```python
from build123d import *

# Parameters (mm, degrees)
SM_BASE_FLANGE_1_DEPTH              = 8
SM_EDGE_FLANGE_1_STRIP_W            = 48
SM_EDGE_FLANGE_1_STRIP_H            = 8
SM_EDGE_FLANGE_1_STRIP_CUT_DEPTH    = 50
SM_EDGE_FLANGE_1_RELIEF_W           = 52
SM_EDGE_FLANGE_1_RELIEF_H           = 4
SM_EDGE_FLANGE_1_RELIEF_CUT_DEPTH   = 8
SM_EDGE_FLANGE_1_STRIP_2_W          = 48
SM_EDGE_FLANGE_1_STRIP_2_H          = 8
SM_EDGE_FLANGE_1_STRIP_CUT_2_DEPTH  = 50
SM_EDGE_FLANGE_1_RELIEF_2_W         = 52
SM_EDGE_FLANGE_1_RELIEF_2_H         = 4
SM_EDGE_FLANGE_1_RELIEF_CUT_2_DEPTH = 8
SM_EDGE_FLANGE_1_DEPTH              = 50
SM_EDGE_FLANGE_1_BEND_DEPTH         = 50


# Sheet-metal steps are written as plain solids
with BuildPart() as part:
    # Sketch 1 → 基体-法兰1 (new body)
    with BuildSketch(Plane(origin=(0, 0, 0), x_dir=(0, 0, -1), z_dir=(1, 0, 0))):
        Polygon((-52.5, 122), (52.5, 122), (114.5, 60), (114.5, 50), (124.5, 50), (124.5, 0), (-124.5, 0), (-124.5, 50), (-114.5, 50), (-114.5, 60), align=None)
    extrude(amount=-SM_BASE_FLANGE_1_DEPTH)

    # 边线-法兰1 strip (across the edge) → 边线-法兰1 strip cut (cut)
    with BuildSketch(Plane(origin=(-8, 0, 124.5), x_dir=(0, 0, -1), z_dir=(0, 1, 0))):
        with Locations((-8, -4)):
            Rectangle(SM_EDGE_FLANGE_1_STRIP_W, SM_EDGE_FLANGE_1_STRIP_H)
    extrude(amount=SM_EDGE_FLANGE_1_STRIP_CUT_DEPTH, mode=Mode.SUBTRACT)

    # 边线-法兰1 relief (on the sheet) → 边线-法兰1 relief cut (cut)
    with BuildSketch(Plane(origin=(-8, 0, 108.5), x_dir=(0, 0, -1), z_dir=(-1, 0, 0))):
        with Locations((-22, -52)):
            Rectangle(SM_EDGE_FLANGE_1_RELIEF_W, SM_EDGE_FLANGE_1_RELIEF_H)
    extrude(amount=-SM_EDGE_FLANGE_1_RELIEF_CUT_DEPTH, mode=Mode.SUBTRACT)

    # 边线-法兰1 strip 2 (across the edge) → 边线-法兰1 strip cut 2 (cut)
    with BuildSketch(Plane(origin=(-8, 50, -124.5), x_dir=(0, 0, 1), z_dir=(0, -1, 0))):
        with Locations((-8, -4)):
            Rectangle(SM_EDGE_FLANGE_1_STRIP_2_W, SM_EDGE_FLANGE_1_STRIP_2_H)
    extrude(amount=SM_EDGE_FLANGE_1_STRIP_CUT_2_DEPTH, mode=Mode.SUBTRACT)

    # 边线-法兰1 relief 2 (on the sheet) → 边线-法兰1 relief cut 2 (cut)
    with BuildSketch(Plane(origin=(-8, 50, -108.5), x_dir=(0, 0, 1), z_dir=(-1, 0, 0))):
        with Locations((-22, 2)):
            Rectangle(SM_EDGE_FLANGE_1_RELIEF_2_W, SM_EDGE_FLANGE_1_RELIEF_2_H)
    extrude(amount=-SM_EDGE_FLANGE_1_RELIEF_CUT_2_DEPTH, mode=Mode.SUBTRACT)

    # 边线-法兰1 section (across the edge) → 边线-法兰1 (add)
    with BuildSketch(Plane(origin=(-8, 0, 124.5), x_dir=(0, 0, -1), z_dir=(0, 1, 0))):
        with BuildLine():
            Line((0, 8), (0, 62))
            Line((0, 62), (8, 62))
            Line((8, 62), (8, 8))
            ThreePointArc((8, 8), (10.343145751, 2.343145751), (16, 0))
            Line((16, 0), (16, -8))
            ThreePointArc((16, -8), (4.686291501, -3.313708499), (0, 8))
        make_face()
    extrude(amount=SM_EDGE_FLANGE_1_DEPTH)

    # 边线-法兰1 section 2 (across the edge) → 边线-法兰1 bend (add)
    with BuildSketch(Plane(origin=(-8, 50, -124.5), x_dir=(0, 0, 1), z_dir=(0, -1, 0))):
        with BuildLine():
            Line((0, 8), (0, 62))
            Line((0, 62), (8, 62))
            Line((8, 62), (8, 8))
            ThreePointArc((8, 8), (10.343145751, 2.343145751), (16, 0))
            Line((16, 0), (16, -8))
            ThreePointArc((16, -8), (4.686291501, -3.313708499), (0, 8))
        make_face()
    extrude(amount=SM_EDGE_FLANGE_1_BEND_DEPTH)


solid = part.part
```
Could you check a few things on this model? Use its own coordinates, in mm. A direction names the side the tool comes from. Round coordinates to 2 decimals unless told otherwise and drop trailing zeros. Write each loop counter-clockwise with the first axis right and the second up, starting at its lowest first coordinate (ties: lowest second). Pieces come first, ordered by that corner, then holes. Notation, with made-up numbers: M -2,-22.75 L 4,-22.75 A21 ccw 4,-1.75 Z; hole C 58,62 d9. An arc over 180 degrees is marked long. Write each question's results on one line, items separated by ' | '. Start each with the question number.
1. I'm going to push flat-ended pins straight in: pin 1 Ø4.5 at (x, y) = (-3, 51.5) entering from -Z; pin 2 Ø12 at (y, z) = (40, -52.5) entering from -X; pin 3 Ø16 at (x, z) = (-30, 117.5) entering from +Y; pin 4 Ø10 at (x, z) = (-10.5, -26.5) entering from -Y. Where does each tip first touch, or does it pass through?
2. Imagine slicing it at C-C on z = -64. List the corners of the cut face in (x, y) for me, and give its area (3 significant figures).
3. Imagine slicing it at B-B on y = 43. List the corners of the cut face in (x, z) for me.
4. I need wall thicknesses on L1, parallel to Z at x = -16, y = 40.5; L2, parallel to X at y = 47, z = -99.5; L3, parallel to Y at x = -7, z = 84.5. Which ranges of each line are inside material? Lowest first, please. Write a range as from..to.
5. On a 3-axis mill with a long thin cutter (end or side, diameter ignored), from which of +Z, -Z, +X, -X, +Y, -Y can I reach the whole of each face in a straight line? I mean faces 1 (the face through (-10.406, 25.35, -114.219)), 2 (the face through (-4.563, 25.35, -119.689)), 3 (the face through (-4, 54, 110)), 4 (the face through (-35, 50, -119)), 5 (the face through (-4, 57, 114.5)). Say none if no direction works.
6. Imagine slicing it at A-A on x = -24. List the corners of the cut face in (y, z) for me, and give its area (3 significant figures).
7. Imagine slicing it at D-D on y = 105. List the corners of the cut face in (x, z) for me.
8. Thinking about a two-plate mould opening in Z: for faces 6 (the face through (0, 62, -2)), 7 (the face through (-43, 25, -116.5)), 8 (the face through (-4.563, 24.65, 119.689)), which applies, +Z half, -Z half, draft (parallel to the pull), parting line (faces both ways), or undercut?
Result sheet:
1) pin 1: stops at z = -119.8 | pin 2: stops at x = -8 | pin 3: stops at y = 50 | pin 4: stops at y = 0
2) outline: M -8,0 L 0,0 L 0,110.5 L -8,110.5 Z | area: 884 mm^2
3) outline: M -70,-124.5 L -16,-124.5 A16 ccw 0,-108.5 L 0,108.5 A16 ccw -16,124.5 L -70,124.5 L -70,116.5 L -16,116.5 A8 cw -8,108.5 L -8,-108.5 A8 cw -16,-116.5 L -70,-116.5 Z
4) L1: z = -124.5..-116.5, 116.5..124.5 | L2: x = -8..0 | L3: y = 0..90
5) face 1: -X, +Y, -Y | face 2: -Z, +X, -Y | face 3: +Z, +X, -X | face 4: -Z, +X, -X | face 5: +Z, +X, -X, +Y
6) outline: M 0,-124.5 L 50,-124.5 L 50,-116.5 L 0,-116.5 Z; M 0,116.5 L 50,116.5 L 50,124.5 L 0,124.5 Z | area: 800 mm^2
7) outline: M -8,-69.5 L 0,-69.5 L 0,69.5 L -8,69.5 Z
8) face 6: draft | face 7: undercut | face 8: +Z half
